Build history of the part. All positions in model axes, mm. A direction names the side the tool comes from. Coordinates: 2 decimals unless noted, no trailing zeros. Write each loop counter-clockwise with the first axis right and the second up, starting at its lowest first coordinate (ties: lowest second). Pieces come first, ordered by that corner, then holes.
from build123d import *

# Parameters (mm, degrees)
F0_W     = 25.536726
F0_H     = 20
F1_DEPTH = 20
F3_DEPTH = 5


with BuildPart() as f1:
    # F0 (on Front) → F1 (new body, symmetric)
    with BuildSketch(Plane.XZ):
        Rectangle(F0_W, F0_H)
    extrude(amount=F1_DEPTH, both=True)

    # F2 (on face) → F3 (cut)
    with BuildSketch(Plane.XZ.offset(20)):
        with BuildLine():
            ThreePointArc((4.863993, 4.458256), (3.609529, 4.863258), (2.375522, 4.399647))
            ThreePointArc((2.375522, 4.399647), (-3.082954, 3.936419), (-4.840709, -1.252014))
            ThreePointArc((-4.840709, -1.252014), (-5.231428, -4.09718), (-2.375531, -4.399642))
            ThreePointArc((-2.375531, -4.399642), (3.082946, -3.936425), (4.840711, 1.252004))
            ThreePointArc((4.840711, 1.252004), (5.585837, 2.336443), (5.495987, 3.649131))
            Line((5.495987, 3.649131), (14.416598, 11.198342))
            Line((14.416598, 11.198342), (14.321596, 11.310602))
            Line((14.321596, 11.310602), (4.863993, 4.458256))
        make_face()
    extrude(amount=-F3_DEPTH, mode=Mode.SUBTRACT)


solid = f1.part
(1) 3-axis set-ups, long thin cutter, end or side, ignore diameter. For faces 1 (the cylindrical face through (5.58, -17.54, 2.32)), 2 (the flat face through (0, 20, 0)): which of +Z, -Z, +X, -X, +Y, -Y reach the whole face in a straight line?
(2) Two-plate mould, pull along X, no slides. Class faces 3 (the cylindrical face through (-3, -18, 4)), 4 (the flat face through (12.768, 0, 0)), 5 (the flat face through (0, 0, -10)): pulls with the +X half, pulls with the -X half, needs draft (parallel to the pull), parting line crosses it, or undercut.
(3) Slice it at C-C, the plane x = -0.75. List the corners of the cut face in (y, z), and give its area (3 significant figures).
(4) Probe L1, parallel to Z at x = 6.5, y = -17.5. List the from-to ranges inside material, lowest first.
(5) Slice it at A-A, the plane z = -3.25. List the corners of the cut face in (x, y).
(6) Slice it at B-B, the plane y = -17. List the corners of the cut face in (x, z), and give its area (3 significant figures).
Results:
1. face 1: -Y
1. face 2: +Z, -Z, +X, -X, +Y
2. face 3: undercut
2. face 4: pulls with the +X half
2. face 5: needs draft
3. outline: (-20, -10) - (20, -10) - (20, 10) - (-20, 10) - (-20, 4.94) - (-15, 4.94) - (-15, -4.94) - (-20, -4.94) - close
3. area: 751 mm2
4. L1: z = -10 to 4.5, 5.64 to 10
5. outline: (-12.77, -20) - (-5.62, -20) - (-5.62, -15) - (3.8, -15) - (3.8, -20) - (12.77, -20) - (12.77, 20) - (-12.77, 20) - close
6. outline: (-12.77, -10) - (12.77, -10) - (12.77, 9.8) - (5.5, 3.65) arc R2 cw to (4.84, 1.25) arc R5 cw to (-2.38, -4.4) arc R2 cw (long way) to (-4.84, -1.25) arc R5 cw to (2.38, 4.4) arc R2 cw to (4.86, 4.46) - (12.51, 10) - (-12.77, 10) - close
6. area: 415 mm2
